Geometry check sheet. Reference: the model listing, model coordinates, mm. Face numbers are marked on the shaded views. A direction names the side the tool comes from. Round coordinates to 2 decimals unless told otherwise and drop trailing zeros. Write each loop counter-clockwise with the first axis right and the second up, starting at its lowest first coordinate (ties: lowest second). Pieces come first, ordered by that corner, then holes. Notation, with made-up numbers: (89, 75.5) -> (106, 75.5) arc R30 ccw to (106, 107.5) -> close; hole circle Ø9 at (53.25, 50). An arc over 180 degrees is marked (long way). Use a Markdown table: item, result.
```python
from build123d import *

# Parameters (mm, degrees)
F0_W     = 127
F0_H     = 127
F1_DEPTH = 50.8
F3_DEPTH = 25.4
F4_DEPTH = 25.4
F5_DEPTH = 25.4
F6_DEPTH = 25.4
F7_DEPTH = 25.4


with BuildPart() as f1:
    # F0 (on Top) → F1 (new body)
    with BuildSketch(Plane.XY):
        with Locations((-1.1648386717, 4.6072422095)):
            Rectangle(F0_W, F0_H)
    extrude(amount=F1_DEPTH)

    # F2 (on face) → F3 (cut)
    with BuildSketch(Plane.XY.offset(50.8)):
        Polygon((11.5351613283, 68.1072422095), (-13.8648386717, 68.1072422095), (-13.8648386717, 17.3072422095), (-64.6648386717, 17.3072422095), (-64.6648386717, -8.0927577905), (-13.8648386717, -8.0927577905), (-13.8648386717, -58.8927577905), (11.5351613283, -58.8927577905), (11.5351613283, -8.0927577905), (62.3351613283, -8.0927577905), (62.3351613283, 17.3072422095), (11.5351613283, 17.3072422095), align=None)
    extrude(amount=-F3_DEPTH, mode=Mode.SUBTRACT)

    # F4 (add): a face of the model
    f4_faces = [f1.faces().sort_by_distance(p)[0] for p in [
        (-1.1648386717, -58.8927577905, 23.9888888889),
    ]]
    extrude(f4_faces, amount=F4_DEPTH)

    # F5 (add): a face of the model
    f5_faces = [f1.faces().sort_by_distance(p)[0] for p in [
        (62.3351613283, -9.247303245, 24.2454545455),
    ]]
    extrude(f5_faces, amount=F5_DEPTH)

    # F6 (add): a face of the model
    f6_faces = [f1.faces().sort_by_distance(p)[0] for p in [
        (12.6897067829, 68.1072422095, 24.2454545455),
    ]]
    extrude(f6_faces, amount=F6_DEPTH)

    # F7 (add): a face of the model
    f7_faces = [f1.faces().sort_by_distance(p)[0] for p in [
        (-64.6648386717, 4.6072422095, 24.4230769231),
    ]]
    extrude(f7_faces, amount=F7_DEPTH)


solid = f1.part
```
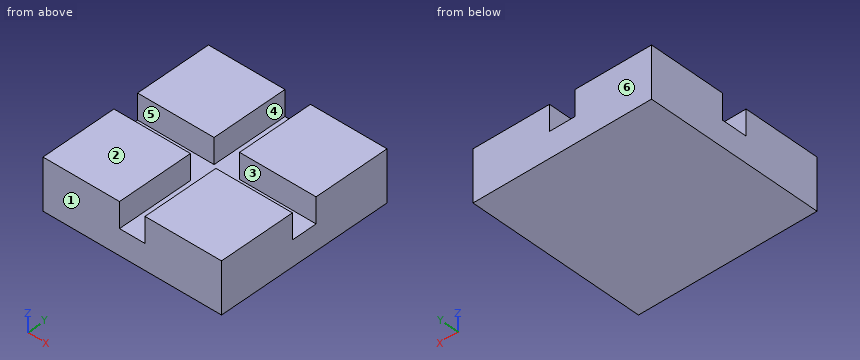
(1) Release check for a two-part mould opening along Y. For the marked faces 1, 2 and 3 record: +Y half, -Y half, draft (parallel to the pull), parting line (faces both ways), or undercut.
A:
| item | result |
|---|---|
| face 1 | -Y half |
| face 2 | draft |
| face 3 | undercut |
(2) Section check B-B on x = 62.5. Record the cut outline in (y, z).
A:
| item | result |
|---|---|
| outline | (-84.29, 0) -> (93.51, 0) -> (93.51, 50.8) -> (17.31, 50.8) -> (17.31, 25.4) -> (-8.09, 25.4) -> (-8.09, 50.8) -> (-84.29, 50.8) -> close |
(3) Thickness scan on line 1 (Y direction, x = 33.5, z = 33); line 2 (X direction, y = 60, z = 38.5); line 3 (Z direction, x = -43, y = 2). Record the ranges inside material, lowest first.
A:
| item | result |
|---|---|
| line 1 | y = -84.29 to -8.09, 17.31 to 93.51 |
| line 2 | x = -90.06 to -13.86, 11.54 to 87.74 |
| line 3 | z = 0 to 25.4 |
(4) Section check A-A on z = 40. Record the cut outline in (x, y).
A:
| item | result |
|---|---|
| outline | (-90.06, -84.29) -> (-13.86, -84.29) -> (-13.86, -8.09) -> (-90.06, -8.09) -> close; (-90.06, 17.31) -> (-13.86, 17.31) -> (-13.86, 93.51) -> (-90.06, 93.51) -> close; (11.54, -84.29) -> (87.74, -84.29) -> (87.74, -8.09) -> (11.54, -8.09) -> close; (11.54, 17.31) -> (87.74, 17.31) -> (87.74, 93.51) -> (11.54, 93.51) -> close |
(5) Section check C-C on y = 48.5. Record the cut outline in (x, z).
A:
| item | result |
|---|---|
| outline | (-90.06, 0) -> (87.74, 0) -> (87.74, 50.8) -> (11.54, 50.8) -> (11.54, 25.4) -> (-13.86, 25.4) -> (-13.86, 50.8) -> (-90.06, 50.8) -> close |
(6) Gauge pin test, flat end, axial feed: pin 1 Ø12 at (x, y) = (-5, 69.5) entering from +Z. Record the tip position at first contact, or that the pin passes through.
A:
| item | result |
|---|---|
| pin 1 | stops at z = 25.4 |
(7) Access from +Z, -Z, +X, -X, +Y, -Y to the whole of each face (thin tool, end or side, straight path). Record for the marked faces 4, 5 and 6.
A:
| item | result |
|---|---|
| face 4 | +Z, +Y, -Y |
| face 5 | +Z, +X, -X |
| face 6 | +Z, -Z, +X, -X, +Y |
(8) Section check D-D on x = -11. Record the cut outline in (y, z).
A:
| item | result |
|---|---|
| outline | (-84.29, 0) -> (93.51, 0) -> (93.51, 25.4) -> (-84.29, 25.4) -> close |
